Build history of the part. All positions in model axes, mm. Give positions to 0.01 mm unless a question says otherwise; leave off trailing zeros. Loops run counter-clockwise (first coordinate to the right, second up) from the corner with the lowest first, then second, coordinate; pieces in that order, holes last.
1) Wall check: line 1 (Z direction, x = 94.6, y = 144); line 2 (Y direction, x = 93.1, z = 1211); line 3 (Y direction, x = 93.7, z = 1172.5). Give the ranges that are in metal, low to high.
2) Band-saw the part on B-B on x = 94.3. State how many separate pieces and enclosed holes the cut face has, then the cut area to 3 significant figures.
3) Band-saw the part on D-D on y = 169.5. List the corners of the cut face in (x, z).
4) Flat gauge pin, fed straight in: P1, Ø1, axis at x = 95, y = 187.5, coming from the +Z side. Where does the tip first touch, or does it go through?
5) Band-saw the part on C-C on z = 1208. List the corners of the cut face in (x, y).
6) Two-plate mould, pull along Y, no slides. Class faces 1 (the flat face through (92.869, 161, 1177)), 2 (the cylindrical face through (94.43, 141.03, 1218.95)), 3 (the cylindrical face through (94.434, 192.784, 1168.467)), 4 (the cylindrical face through (94.434, 200.854, 1162.381)): +Y half, -Y half, draft (parallel to the pull), parting line (faces both ways), or undercut.
7) Band-saw the part on A-A on y = 144. List the corners of the cut face in (x, z), then the cut area to 3 significant figures.
```python
from build123d import *

# Parameters (mm, degrees)
BOSS_EXTRUDE1_START     = 92.868812
BOSS_EXTRUDE1_DEPTH     = 3.175
F_1_4_CLEARANCE_HOLE1_D = 6.7564


with BuildPart() as part:
    # Sketch1 → Boss-Extrude1 (new body)
    with BuildSketch(Plane(origin=(0, 0, 0), x_dir=(0, 0, -1), z_dir=(1, 0, 0)).offset(BOSS_EXTRUDE1_START)):
        with BuildLine():
            Line((-1155.791403712, 192.93801872), (-1149.996384364, 146.073482729))
            ThreePointArc((-1149.996384364, 146.073482729), (-1152.312880663, 138.596176396), (-1159.44938805, 135.379574554))
            Line((-1159.44938805, 135.379574554), (-1210.24938805, 135.379574554))
            ThreePointArc((-1210.24938805, 135.379574554), (-1219.012005401, 141.170654074), (-1217.119501727, 151.502086438))
            Line((-1217.119501727, 151.502086438), (-1172.114521075, 198.366622429))
            ThreePointArc((-1172.114521075, 198.366622429), (-1162.238535685, 200.807382517), (-1155.791403712, 192.93801872))
        make_face()
    extrude(amount=BOSS_EXTRUDE1_DEPTH)

    # 1/4 Clearance Hole1 (through all)
    with Locations(Plane(origin=(96.043812484, 0, 0), x_dir=(0, 0, -1), z_dir=(1, 0, 0))):
        with Locations((-1175.046897724, 168.336842549), (-1165.244407398, 191.769110545), (-1210.24938805, 144.904574554), (-1184.84938805, 144.904574554), (-1159.44938805, 144.904574554)):
            Hole(F_1_4_CLEARANCE_HOLE1_D / 2)


solid = part.part
```
Findings below:
1. line 1: z = 1149.97 to 1156.19, 1162.7 to 1181.59, 1188.1 to 1206.99, 1213.5 to 1219.73
1. line 2: y = 135.41 to 141.61, 148.2 to 157.87
1. line 3: y = 135.38 to 166.12, 170.56 to 197.97
2. separate pieces: 1
2. enclosed holes: 5
2. area: 2,850 mm2
3. outline: (92.87, 1152.89) - (96.04, 1152.89) - (96.04, 1171.88) - (92.87, 1171.88) - close; (92.87, 1178.22) - (96.04, 1178.22) - (96.04, 1199.84) - (92.87, 1199.84) - close
4. P1: stops at z = 1183.03
5. outline: (92.87, 135.38) - (96.04, 135.38) - (96.04, 142.38) - (92.87, 142.38) - close; (92.87, 147.42) - (96.04, 147.42) - (96.04, 161) - (92.87, 161) - close
6. face 1: draft
6. face 2: parting line
6. face 3: undercut
6. face 4: +Y half
7. outline: (92.87, 1149.97) - (96.04, 1149.97) - (96.04, 1156.19) - (92.87, 1156.19) - close; (92.87, 1162.7) - (96.04, 1162.7) - (96.04, 1181.59) - (92.87, 1181.59) - close; (92.87, 1188.1) - (96.04, 1188.1) - (96.04, 1206.99) - (92.87, 1206.99) - close; (92.87, 1213.5) - (96.04, 1213.5) - (96.04, 1219.73) - (92.87, 1219.73) - close
7. area: 159 mm2
